Read the model definition and answer for the solid it produces. Units are mm, in the model's axes. A direction names the side the tool comes from. Coordinates: 2 decimals unless noted, no trailing zeros. Write each loop counter-clockwise with the first axis right and the second up, starting at its lowest first coordinate (ties: lowest second). Pieces come first, ordered by that corner, then holes. Notation, with made-up numbers: (52.5, 19.25) -> (65.5, 19.25) arc R20 cw to (65.5, 57.25) -> close; hole circle Ø4 at (52.25, -34). An arc over 180 degrees is marked (long way). One line per item, written item: value. Start each with the question number.
from build123d import *

# Parameters (mm, degrees)
SKETCH1_W           = 300
SKETCH1_H           = 420
BOSS_EXTRUDE1_DEPTH = 6.35
SKETCH3_R           = 3.25
CUT_EXTRUDE1_DEPTH  = 517.178576173
SKETCH4_R           = 2.5
CUT_EXTRUDE2_DEPTH  = 517.178576173
SKETCH6_R           = 1.7
CUT_EXTRUDE3_DEPTH  = 517.178576173
CUT_EXTRUDE4_DEPTH  = 10
SKETCH8_R           = 13.335
CUT_EXTRUDE5_DEPTH  = 517.178576173
SKETCH9_R           = 2.1
CUT_EXTRUDE6_DEPTH  = 517.178576173
CUT_EXTRUDE7_DEPTH  = 517.178576173


with BuildPart() as part:
    # Sketch1 → Boss-Extrude1 (new body)
    with BuildSketch(Plane(origin=(0, 0, 0), x_dir=(1, 0, 0), z_dir=(0, 1, 0))):
        with Locations((150, 210)):
            Rectangle(SKETCH1_W, SKETCH1_H)
    extrude(amount=BOSS_EXTRUDE1_DEPTH)

    # Sketch3 → Cut-Extrude1 (cut, through all)
    with BuildSketch(Plane(origin=(0, 6.35, 0), x_dir=(1, 0, 0), z_dir=(0, 1, 0))):
        with Locations(Location((50, 12.5, 0), (0, 0, 270))):
            Circle(SKETCH3_R)
        with Locations(Location((250, 12.5, 0), (0, 0, 270))):
            Circle(SKETCH3_R)
        with Locations(Location((12.5, 50, 0), (0, 0, 270))):
            Circle(SKETCH3_R)
        with Locations(Location((12.5, 250, 0), (0, 0, 270))):
            Circle(SKETCH3_R)
        with Locations(Location((250, 287.5, 0), (0, 0, 90))):
            Circle(SKETCH3_R)
        with Locations(Location((50, 287.5, 0), (0, 0, 90))):
            Circle(SKETCH3_R)
        with Locations(Location((287.5, 250, 0), (0, 0, 90))):
            Circle(SKETCH3_R)
        with Locations(Location((287.5, 50, 0), (0, 0, 90))):
            Circle(SKETCH3_R)
    extrude(amount=-CUT_EXTRUDE1_DEPTH, mode=Mode.SUBTRACT)

    # Sketch4 → Cut-Extrude2 (cut, through all)
    with BuildSketch(Plane(origin=(0, 6.35, 0), x_dir=(1, 0, 0), z_dir=(0, 1, 0))):
        with Locations(Location((20.55, 12.5, 0), (0, 0, 270))):
            Circle(SKETCH4_R)
        with Locations(Location((274.55, 12.5, 0), (0, 0, 270))):
            Circle(SKETCH4_R)
        with Locations(Location((20.55, 387.5, 0), (0, 0, 270))):
            Circle(SKETCH4_R)
        with Locations(Location((274.55, 387.5, 0), (0, 0, 270))):
            Circle(SKETCH4_R)
    extrude(amount=-CUT_EXTRUDE2_DEPTH, mode=Mode.SUBTRACT)

    # Sketch6 → Cut-Extrude3 (cut, through all)
    with BuildSketch(Plane(origin=(0, 6.35, 0), x_dir=(1, 0, 0), z_dir=(0, 1, 0))):
        with Locations(Location((282.5, 355, 0), (0, 0, 270))):
            Circle(SKETCH6_R)
        with Locations(Location((100, 336, 0), (0, 0, 270))):
            Circle(SKETCH6_R)
        with Locations(Location((100, 374, 0), (0, 0, 270))):
            Circle(SKETCH6_R)
    extrude(amount=-CUT_EXTRUDE3_DEPTH, mode=Mode.SUBTRACT)

    # Sketch7 → Cut-Extrude4 (cut)
    with BuildSketch(Plane(origin=(0, 6.35, 0), x_dir=(1, 0, 0), z_dir=(0, 1, 0))):
        with BuildLine():
            Line((290, 420), (300, 420))
            Line((300, 420), (300, 410))
            ThreePointArc((300, 410), (297.071067812, 417.071067812), (290, 420))
        make_face()
        with BuildLine():
            Line((10, 420), (0, 420))
            Line((0, 420), (0, 410))
            ThreePointArc((0, 410), (2.928932188, 417.071067812), (10, 420))
        make_face()
    extrude(amount=-CUT_EXTRUDE4_DEPTH, mode=Mode.SUBTRACT)

    # Sketch8 → Cut-Extrude5 (cut, through all)
    with BuildSketch(Plane(origin=(0, 6.35, 0), x_dir=(1, 0, 0), z_dir=(0, 1, 0))):
        with Locations(Location((70, 335, 0), (0, 0, 270))):
            Circle(SKETCH8_R)
        with Locations(Location((30, 335, 0), (0, 0, 270))):
            Circle(SKETCH8_R)
    extrude(amount=-CUT_EXTRUDE5_DEPTH, mode=Mode.SUBTRACT)

    # Sketch9 → Cut-Extrude6 (cut, through all)
    with BuildSketch(Plane(origin=(0, 6.35, 0), x_dir=(1, 0, 0), z_dir=(0, 1, 0))):
        with Locations(Location((282.5, 324, 0), (0, 0, 270))):
            Circle(SKETCH9_R)
        with Locations(Location((111, 405, 0), (0, 0, 270))):
            Circle(SKETCH9_R)
        with Locations(Location((113, 324, 0), (0, 0, 270))):
            Circle(SKETCH9_R)
    extrude(amount=-CUT_EXTRUDE6_DEPTH, mode=Mode.SUBTRACT)

    # Sketch10 → Cut-Extrude7 (cut, through all)
    with BuildSketch(Plane(origin=(0, 6.35, 0), x_dir=(1, 0, 0), z_dir=(0, 1, 0))):
        with BuildLine():
            Line((55, 25), (35, 25))
            ThreePointArc((35, 25), (25, 35), (35, 45))
            Line((35, 45), (55, 45))
            ThreePointArc((55, 45), (65, 35), (55, 25))
        make_face()
    extrude(amount=-CUT_EXTRUDE7_DEPTH, mode=Mode.SUBTRACT)


solid = part.part
1. Find the intervals of material crossed by probe 1 along Z at (x, y) = (100, 1.75); probe 2 along Z at (x, y) = (287.5, 5); probe 3 along X at (y, z) = (1.5, -336), in increasing order. Write a range as from..to.
2. For a pull along X with two mould halves and no side action, classify faces 1 (the face through (148, 0, -213)), 2 (the face through (297.15, 3.22, -416.99)), 3 (the face through (25, 3, -35)) as +X half, -X half, draft (parallel to the pull), parting line (faces both ways), or undercut.
3. Given pin 1 (3 mm diameter, centred on x = 282.5, z = -355, fed in from -Y), flat-ended and moving along its own axis, determine where the tip first touches the part or whether it passes through.
4. A cutting plane is placed at B-B on z = -36. Give the vertices of the cut face in (x, y).
5. A cutting plane is placed at A-A on y = 5. Count the separate pieces of the cut face and the enclosed holes in it, then the cut area to 3 significant figures.
6. A tool of negligible diameter and unlimited length cuts with its end or side. For faces 4 (the face through (65, 3, -35)), 5 (the face through (2.85, 3.22, -416.99)), from which of +Z, -Z, +X, -X, +Y, -Y can it reach the whole face along a straight path? Write none if from no direction.
Derived:
1. probe 1: z = -420..-375.7, -372.3..-337.7, -334.3..0
1. probe 2: z = -420..-253.25, -246.75..-53.25, -46.75..0
1. probe 3: x = 0..16.7, 43.3..56.7, 83.3..98.3, 101.7..300
2. face 1: draft
2. face 2: +X half
2. face 3: undercut
3. pin 1: passes through
4. outline: (0, 0) -> (25.05, 0) -> (25.05, 6.35) -> (0, 6.35) -> close; (64.95, 0) -> (300, 0) -> (300, 6.35) -> (64.95, 6.35) -> close
5. separate pieces: 1
5. enclosed holes: 21
5. area: 124,000 mm2
6. face 4: +Y, -Y
6. face 5: -Z, -X, +Y, -Y
